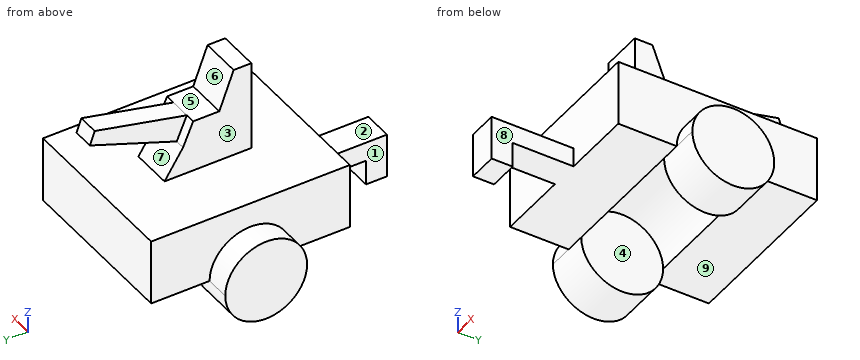
```python
from build123d import *

# Parameters (mm, degrees)
F1_DEPTH = 36.83
F2_DEPTH = 47.498
F3_DEPTH = 28.194
F4_DEPTH = 8.89
F5_DEPTH = 4.572
F6_DEPTH = 6.35
F7_W     = 33.954457
F7_H     = 11.318151
F8_DEPTH = 12.7


with BuildPart() as f1:
    # F0 (on Right) → F1 (new body, symmetric)
    with BuildSketch(Plane.YZ):
        with BuildLine():
            Line((-18.119462, 14.21879), (-42.990837, 14.21879))
            Line((-42.990837, 14.21879), (-42.990837, -5.931014))
            Line((-42.990837, -5.931014), (-42.990837, -14.21879))
            Line((-42.990837, -14.21879), (-17.70777, -14.21879))
            ThreePointArc((-17.70777, -14.21879), (0, 3.48898), (17.70777, -14.21879))
            Line((17.70777, -14.21879), (42.990837, -14.21879))
            Line((42.990837, -14.21879), (42.990837, 14.21879))
            Line((42.990837, 14.21879), (19.459361, 14.21879))
            Line((19.459361, 14.21879), (-18.119462, 14.21879))
        make_face()
    extrude(amount=F1_DEPTH, both=True)

    # F0 (on Right) → F2 (join, symmetric)
    with BuildSketch(Plane.YZ):
        with BuildLine():
            ThreePointArc((17.70777, -14.21879), (0, 3.48898), (-17.70777, -14.21879))
            ThreePointArc((-17.70777, -14.21879), (0, -31.926559), (17.70777, -14.21879))
        make_face()
    extrude(amount=F2_DEPTH, both=True)

    # F0 (on Right) → F3 (cut, symmetric)
    with BuildSketch(Plane.YZ):
        with BuildLine():
            ThreePointArc((17.70777, -14.21879), (0, 3.48898), (-17.70777, -14.21879))
            ThreePointArc((-17.70777, -14.21879), (0, -31.926559), (17.70777, -14.21879))
        make_face()
    extrude(amount=F3_DEPTH, both=True, mode=Mode.SUBTRACT)

    # F0 (on Right) → F4 (join, symmetric)
    with BuildSketch(Plane.YZ):
        Polygon((-18.119462, 53.173751), (-18.119462, 14.21879), (19.459361, 14.21879), (11.432814, 26.540214), (7.054701, 36.755815), (-4.25543, 36.755815), (-10.457761, 53.173751), align=None)
    extrude(amount=F4_DEPTH, both=True)

    # F0 (on Right) → F5 (join, symmetric)
    with BuildSketch(Plane.YZ):
        Polygon((7.054701, 36.755815), (11.432814, 26.540214), (49.011637, 40.039402), (46.927817, 45.840306), align=None)
    extrude(amount=F5_DEPTH, both=True)

    # F0 (on Right) → F6 (join, symmetric)
    with BuildSketch(Plane.YZ):
        Polygon((-42.990837, -14.21879), (-42.990837, -5.931014), (-78.437544, -5.931014), (-78.437544, -14.21879), (-69.339758, -14.21879), align=None)
        Polygon((-69.339758, -31.358585), (-69.339758, -14.21879), (-78.437544, -14.21879), (-78.437544, -31.283986), align=None)
    extrude(amount=F6_DEPTH, both=True)

    # F7 (on Right) → F8 (cut, symmetric)
    with BuildSketch(Plane.YZ):
        with Locations((-71.897797, -30.766496)):
            Rectangle(F7_W, F7_H)
    extrude(amount=F8_DEPTH, both=True, mode=Mode.SUBTRACT)


solid = f1.part
```
Design review of the part built by this model. Coordinates are the model's own, in mm. Face numbers are marked on the shaded views. A direction names the side the tool comes from. Give positions to 0.01 mm unless a question says otherwise; leave off trailing zeros. Loops run counter-clockwise (first coordinate to the right, second up) from the corner with the lowest first, then second, coordinate; pieces in that order, holes last. Notation, with made-up numbers: M 15,88.5 L 22,88.5 A6 cw 22,92.5 Z; hole C 55,80 d1. An arc over 180 degrees is marked long. Return JSON: item names as keys, results as strings. Group by question number.
Item 1: We need section A-A (z = 42). Give the boundary of the cut face in (x, y), and give its area (3 significant figures).
Item 2: We need section B-B (y = 0). Give the boundary of the cut face in (x, z), and give its area (3 significant figures).
Item 3: Insertion check: pin 1 Ø12 at (x, z) = (-28.5, -15.5) entering from -Y; pin 2 Ø5 at (x, y) = (12, 14) entering from +Z; pin 3 Ø8 at (x, z) = (34.5, 5.5) entering from +Y; pin 4 Ø22 at (x, y) = (-11.5, -13.5) entering from +Z. Each pin has a flat end and moves straight along its axis. Give the tip position at first contact, or say it passes through.
Item 4: Tool access review of the marked faces 1, 2, 3, 4 and 5: name each direction out of +Z, -Z, +X, -X, +Y, -Y from which nothing blocks a thin tool from reaching the whole face with its end or side.
Item 5: We need section D-D (z = 0). Give the boundary of the cut face in (x, y).
Item 6: Mouldability with a two-part tool opening along Z and no side actions: class the marked faces 6, 7, 8 and 9 as released by +Z, released by -Z, zero draft, split by the parting line, or undercut.
Item 7: We need section C-C (y = 15). Give the boundary of the cut face in (x, z), and give its area (3 significant figures).
Item 8: For probe 1 along X at (y, z) = (3.5, -9); probe 2 along Z at (x, y) = (-27, 35); probe 3 along X at (y, z) = (14.5, 20), list the stretches that pass through material, from the lowest coordinate up.
Output:
{
 "1": {"outline": "M -8.89,-18.12 L 8.89,-18.12 L 8.89,-6.24 L -8.89,-6.24 Z; M -4.57,30.07 L 4.57,30.07 L 4.57,48.31 L -4.57,48.31 Z", "area": "378 mm^2"},
 "2": {"outline": "M -47.5,-31.93 L -28.19,-31.93 L -28.19,3.49 L 28.19,3.49 L 28.19,-31.93 L 47.5,-31.93 L 47.5,3.49 L 36.83,3.49 L 36.83,14.22 L 8.89,14.22 L 8.89,36.76 L -8.89,36.76 L -8.89,14.22 L -36.83,14.22 L -36.83,3.49 L -47.5,3.49 Z", "area": "2,560 mm^2"},
 "3": {"pin 1": "stops at y = -42.99", "pin 2": "stops at z = 14.22", "pin 3": "stops at y = 42.99", "pin 4": "stops at z = 53.17"},
 "4": {"face 1": "+Z, -Z, -X, -Y", "face 2": "+Z, +X, -X, -Y", "face 3": "+Z, -X, +Y, -Y", "face 4": "-Z", "face 5": "+Z, +X, -X"},
 "5": {"outline": "M -47.5,-10.55 L -36.83,-10.55 L -36.83,-42.99 L 36.83,-42.99 L 36.83,-10.55 L 47.5,-10.55 L 47.5,10.55 L 36.83,10.55 L 36.83,42.99 L -36.83,42.99 L -36.83,10.55 L -47.5,10.55 Z; hole M -28.19,-10.55 L 28.19,-10.55 L 28.19,10.55 L -28.19,10.55 Z"},
 "6": {"face 6": "released by +Z", "face 7": "undercut", "face 8": "zero draft", "face 9": "released by -Z"},
 "7": {"outline": "M -47.5,-23.63 L -28.19,-23.63 L -28.19,-4.81 L 28.19,-4.81 L 28.19,-23.63 L 47.5,-23.63 L 47.5,-4.81 L 36.83,-4.81 L 36.83,14.22 L 8.89,14.22 L 8.89,21.06 L -8.89,21.06 L -8.89,14.22 L -36.83,14.22 L -36.83,-4.81 L -47.5,-4.81 Z; M -4.57,27.82 L 4.57,27.82 L 4.57,38.57 L -4.57,38.57 Z", "area": "2,350 mm^2"},
 "8": {"probe 1": "x = -47.5 to -28.19, 28.19 to 47.5", "probe 2": "z = -14.22 to 14.22", "probe 3": "x = -8.89 to 8.89"}
}
